from build123d import *

# Parameters (mm, degrees)
EXTRUDE_THIN1_DEPTH      = 34.925
EXTRUDE_THIN1_DEPTH_BACK = 1
EXTRUDE_THIN2_START      = -1
EXTRUDE_THIN2_DEPTH      = 1
FILLET1_R                = 1
SKETCH2_R                = 0.875
CUT_EXTRUDE1_DEPTH       = 6
MIRROR2_COPY_1_SKETCH_R  = 0.875
MIRROR2_COPY_1_DEPTH     = 6
CUT_EXTRUDE2_REACH       = 160.855
SKETCH3_R                = 3.6
CUT_EXTRUDE3_REACH       = 162.855
CUT_EXTRUDE3_START       = -2
SKETCH4_R                = 5.8
SKETCH5_R                = 0.9
CUT_EXTRUDE4_DEPTH       = 4


with BuildPart() as part:
    # Sketch1 → Extrude-Thin1 (new, two sides: drawn at the far end of the back side and taken through both)
    with BuildSketch(Plane(origin=(0, 0, 0), x_dir=(0, 0, -1), z_dir=(1, 0, 0)).offset(-EXTRUDE_THIN1_DEPTH_BACK)):
        with BuildLine():
            Line((72.46875, -37.1475), (72.46875, 37.1475))
            ThreePointArc((72.46875, 37.1475), (67.284540027, 49.663290027), (54.76875, 54.8475))
            Line((54.76875, 54.8475), (-54.76875, 54.8475))
            ThreePointArc((-54.76875, 54.8475), (-67.284540027, 49.663290027), (-72.46875, 37.1475))
            Line((-72.46875, 37.1475), (-72.46875, -37.1475))
            ThreePointArc((-72.46875, -37.1475), (-67.284540027, -49.663290027), (-54.76875, -54.8475))
            Line((-54.76875, -54.8475), (54.76875, -54.8475))
            ThreePointArc((54.76875, -54.8475), (67.284540027, -49.663290027), (72.46875, -37.1475))
        make_face()
        with BuildLine():
            Line((67.46875, -37.1475), (67.46875, 37.1475))
            ThreePointArc((67.46875, 37.1475), (63.749006121, 46.127756121), (54.76875, 49.8475))
            Line((54.76875, 49.8475), (-54.76875, 49.8475))
            ThreePointArc((-54.76875, 49.8475), (-63.749006121, 46.127756121), (-67.46875, 37.1475))
            Line((-67.46875, 37.1475), (-67.46875, -37.1475))
            ThreePointArc((-67.46875, -37.1475), (-63.749006121, -46.127756121), (-54.76875, -49.8475))
            Line((-54.76875, -49.8475), (54.76875, -49.8475))
            ThreePointArc((54.76875, -49.8475), (63.749006121, -46.127756121), (67.46875, -37.1475))
        make_face(mode=Mode.SUBTRACT)
    extrude(amount=EXTRUDE_THIN1_DEPTH + EXTRUDE_THIN1_DEPTH_BACK)

    # Sketch1<2> → Extrude-Thin2 (add)
    with BuildSketch(Plane(origin=(0, 0, 0), x_dir=(0, 0, -1), z_dir=(1, 0, 0)).offset(EXTRUDE_THIN2_START)):
        with BuildLine():
            Line((67.46875, -37.1475), (67.46875, 37.1475))
            ThreePointArc((67.46875, 37.1475), (63.749006121, 46.127756121), (54.76875, 49.8475))
            Line((54.76875, 49.8475), (-54.76875, 49.8475))
            ThreePointArc((-54.76875, 49.8475), (-63.749006121, 46.127756121), (-67.46875, 37.1475))
            Line((-67.46875, 37.1475), (-67.46875, -37.1475))
            ThreePointArc((-67.46875, -37.1475), (-63.749006121, -46.127756121), (-54.76875, -49.8475))
            Line((-54.76875, -49.8475), (54.76875, -49.8475))
            ThreePointArc((54.76875, -49.8475), (63.749006121, -46.127756121), (67.46875, -37.1475))
        make_face()
        with BuildLine():
            Line((61.46875, -37.1475), (61.46875, 37.1475))
            ThreePointArc((61.46875, 37.1475), (59.506365434, 41.885115434), (54.76875, 43.8475))
            Line((54.76875, 43.8475), (-54.76875, 43.8475))
            ThreePointArc((-54.76875, 43.8475), (-59.506365434, 41.885115434), (-61.46875, 37.1475))
            Line((-61.46875, 37.1475), (-61.46875, -37.1475))
            ThreePointArc((-61.46875, -37.1475), (-59.506365434, -41.885115434), (-54.76875, -43.8475))
            Line((-54.76875, -43.8475), (54.76875, -43.8475))
            ThreePointArc((54.76875, -43.8475), (59.506365434, -41.885115434), (61.46875, -37.1475))
        make_face(mode=Mode.SUBTRACT)
    extrude(amount=EXTRUDE_THIN2_DEPTH)

    # Fillet1
    fillet1_edges = [part.edges().sort_by_distance(p)[0] for p in [
        (-1, -49.663290027, -67.284540027),
        (-1, -54.8475, 0),
        (-1, -49.663290027, 67.284540027),
        (-1, 0, 72.46875),
        (-1, 49.663290027, 67.284540027),
        (-1, 54.8475, 0),
        (-1, 49.663290027, -67.284540027),
        (-1, 0, -72.46875),
        (-1, -41.885115434, -59.506365434),
        (-1, -43.8475, 0),
        (-1, -41.885115434, 59.506365434),
        (-1, 0, 61.46875),
        (-1, 41.885115434, 59.506365434),
        (-1, 43.8475, 0),
        (-1, 41.885115434, -59.506365434),
        (-1, 0, -61.46875),
        (0, 49.8475, 0),
        (0, 46.127756121, -63.749006121),
        (0, 0, -67.46875),
        (0, -46.127756121, -63.749006121),
        (0, -49.8475, 0),
        (0, -46.127756121, 63.749006121),
        (0, 0, 67.46875),
        (0, 46.127756121, 63.749006121),
    ]]
    fillet(fillet1_edges, radius=FILLET1_R - 0.0001)  # a hair under: the kernel refuses the full size

    # Sketch2 → Cut-Extrude1 (cut)
    with BuildSketch(Plane(origin=(34.925, 0, 0), x_dir=(0, 0, -1), z_dir=(1, 0, 0))):
        with Locations((69.96875, -37.1475)):
            Circle(SKETCH2_R)
        with Locations((69.96875, -12.3825)):
            Circle(SKETCH2_R)
        with Locations((54.76875, -52.3475)):
            Circle(SKETCH2_R)
        with Locations((10.95375, -52.3475)):
            Circle(SKETCH2_R)
        with Locations((32.86125, -52.3475)):
            Circle(SKETCH2_R)
    cut_extrude1 = extrude(amount=-CUT_EXTRUDE1_DEPTH, mode=Mode.SUBTRACT)

    # Mirror1: Cut-Extrude1 across plane
    add(cut_extrude1.mirror(Plane.XY), mode=Mode.SUBTRACT)

    # Mirror2: Cut-Extrude1 across plane
    add(cut_extrude1.mirror(Plane.ZX), mode=Mode.SUBTRACT)

    # Mirror2 copy 1 sketch → Mirror2 copy 1 (cut)
    with BuildSketch(Plane(origin=(34.925, 0, 0), x_dir=(0, 0, 1), z_dir=(1, 0, 0))):
        with Locations((69.96875, -37.1475)):
            Circle(MIRROR2_COPY_1_SKETCH_R)
        with Locations((69.96875, -12.3825)):
            Circle(MIRROR2_COPY_1_SKETCH_R)
        with Locations((54.76875, -52.3475)):
            Circle(MIRROR2_COPY_1_SKETCH_R)
        with Locations((10.95375, -52.3475)):
            Circle(MIRROR2_COPY_1_SKETCH_R)
        with Locations((32.86125, -52.3475)):
            Circle(MIRROR2_COPY_1_SKETCH_R)
    extrude(amount=-MIRROR2_COPY_1_DEPTH, mode=Mode.SUBTRACT)

    # Sketch3 → Cut-Extrude2 (cut, up to next)
    with BuildSketch(Plane.XY.offset(72.46875), mode=Mode.PRIVATE) as cut_extrude2_sk1:
        with Locations((19.925, 25.1475)):
            Circle(SKETCH3_R)
    cut_extrude2_tool1 = extrude(cut_extrude2_sk1.sketch, amount=-CUT_EXTRUDE2_REACH, mode=Mode.PRIVATE) & part.part
    add(cut_extrude2_tool1.solids().sort_by_distance((19.925, 25.1475, 72.46875))[0], mode=Mode.SUBTRACT)

    # Sketch4 → Cut-Extrude3 (cut, up to next)
    with BuildSketch(Plane.XY.offset(72.46875).offset(CUT_EXTRUDE3_START), mode=Mode.PRIVATE) as cut_extrude3_sk1:
        with Locations((19.925, 25.1475)):
            Circle(SKETCH4_R)
    cut_extrude3_tool1 = extrude(cut_extrude3_sk1.sketch, amount=-CUT_EXTRUDE3_REACH, mode=Mode.PRIVATE) & part.part
    add(cut_extrude3_tool1.solids().sort_by_distance((19.925, 25.1475, 70.46875))[0], mode=Mode.SUBTRACT)

    # Sketch5 → Cut-Extrude4 (cut)
    with BuildSketch(Plane(origin=(0, 0, 67.46875), x_dir=(-1, 0, 0), z_dir=(0, 0, -1))):
        with Locations(Location((-19.925, 35.1475, 0), (0, 0, 90))):
            Circle(SKETCH5_R)
        with Locations(Location((-19.925, 15.1475, 0), (0, 0, 90))):
            Circle(SKETCH5_R)
    extrude(amount=-CUT_EXTRUDE4_DEPTH, mode=Mode.SUBTRACT)


solid = part.part
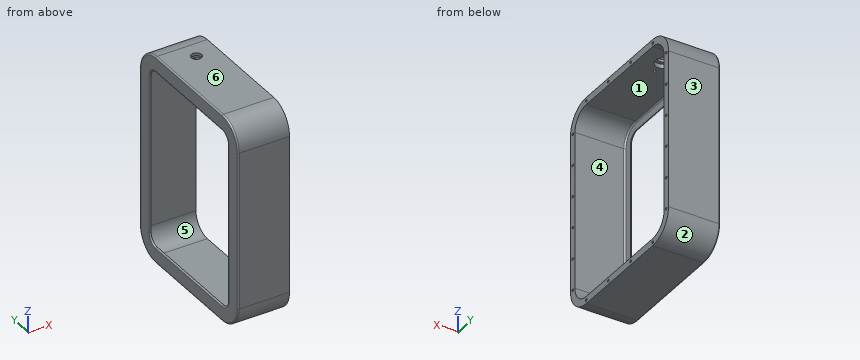
Read the model definition and answer for the solid it produces. Units are mm, in the model's axes. Face numbers are marked on the shaded views. A direction names the side the tool comes from. Give positions to 0.01 mm unless a question says otherwise; leave off trailing zeros. Loops run counter-clockwise (first coordinate to the right, second up) from the corner with the lowest first, then second, coordinate; pieces in that order, holes last. Notation, with made-up numbers: (36.5, 29) -> (90.5, 29) arc R15 cw to (90.5, 38) -> close; hole circle Ø2 at (77, -5.5). An arc over 180 degrees is marked (long way). Use a Markdown table: item, result.
Q1. A tool of negligible diameter and unlimited length cuts with its end or side. For the marked faces 5 and 6, from which of +Z, -Z, +X, -X, +Y, -Y can it reach the whole face along a straight path? Write none if from no direction.
Solved:
| item | result |
|---|---|
| face 5 | +X |
| face 6 | +Z, +X, -X, +Y, -Y |
Q2. Find the intervals of material crossed by line 1 along Y through (x, z) = (33, -37); line 2 along Z through (x, y) = (15, 13.5); line 3 along Z through (x, y) = (29, -46), in increasing order.
Solved:
| item | result |
|---|---|
| line 1 | y = -54.85 to -49.85, 49.85 to 54.85 |
| line 2 | z = -72.47 to -67.47, 67.47 to 72.47 |
| line 3 | z = -70.1 to -63.87, 63.87 to 70.1 |
Q3. Section C-C, the plane x = 9 is taken. Determine the outline of the cut face in (y, z), then the cut area to 3 significant figures.
Solved:
| item | result |
|---|---|
| outline | (-54.85, -54.77) arc R17.7 ccw to (-37.15, -72.47) -> (37.15, -72.47) arc R17.7 ccw to (54.85, -54.77) -> (54.85, 54.77) arc R17.7 ccw to (37.15, 72.47) -> (-37.15, 72.47) arc R17.7 ccw to (-54.85, 54.77) -> close; hole (-49.85, -54.77) arc R12.7 ccw to (-37.15, -67.47) -> (37.15, -67.47) arc R12.7 ccw to (49.85, -54.77) -> (49.85, 54.77) arc R12.7 ccw to (37.15, 67.47) -> (-37.15, 67.47) arc R12.7 ccw to (-49.85, 54.77) -> close |
| area | 2,320 mm^2 |
Q4. Each of these flat-tipped pins is pushed along its axis until it touches: pin 1 (0.5 mm diameter, centred on y = -12.5, z = 70, fed in from +X) (3 decimals); pin 2 (12 mm diameter, centred on x = 22, y = 23, fed in from +Z); pin 3 (5 mm diameter, centred on x = 16.5, y = -40.5, fed in from +Z). Where does it stop, or does it pass through?
Solved:
| item | result |
|---|---|
| pin 1 | stops at x = 28.925 |
| pin 2 | stops at z = 72.47 |
| pin 3 | stops at z = 72.45 |
Q5. Determine the mould class of the marked faces 1, 2, 3 and 4 for opening direction Z: pulls with the +Z half, pulls with the -Z half, needs draft (parallel to the pull), parting line crosses it, or undercut.
Solved:
| item | result |
|---|---|
| face 1 | undercut |
| face 2 | pulls with the -Z half |
| face 3 | needs draft |
| face 4 | undercut |
